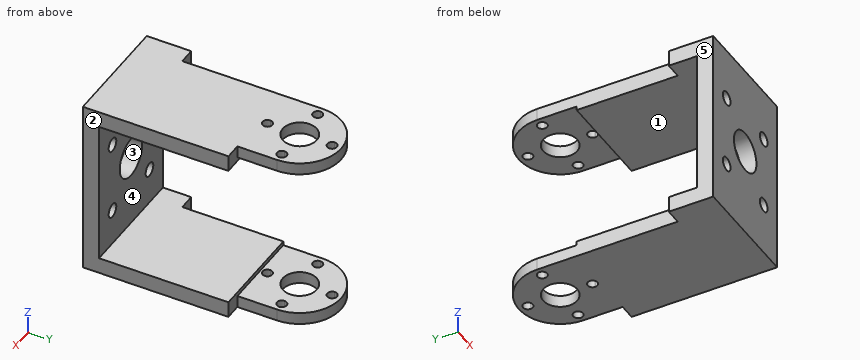
```python
from build123d import *

# Parameters (mm, degrees)
BOSS_EXTRUDE1_DEPTH      = 22
BOSS_EXTRUDE1_DEPTH_BACK = 22
SKETCH2_W                = 38
SKETCH2_H                = 20
CUT_EXTRUDE1_DEPTH       = 105.423416914
SKETCH3_W                = 7
SKETCH3_H                = 44
BOSS_EXTRUDE2_DEPTH      = 36
SKETCH5_W                = 34
SKETCH5_H                = 50
CUT_EXTRUDE3_DEPTH       = 109.047443283
SKETCH6_W                = 20.5
SKETCH6_H                = 54.25
CUT_EXTRUDE4_DEPTH       = 111.605436123
SKETCH20_W               = 28.5
SKETCH20_H               = 34
SKETCH20_R               = 1.7
SKETCH20_R_2             = 5
BOSS_EXTRUDE5_DEPTH      = 4
SKETCH21_W               = 3
SKETCH21_H               = 36
CUT_EXTRUDE12_DEPTH      = 66.777085676
SKETCH22_W               = 4
SKETCH22_H               = 25
CUT_EXTRUDE14_DEPTH      = 66.054784605
CUT_EXTRUDE15_DEPTH      = 57.367654732
CUT_EXTRUDE15_DEPTH_BACK = 57.367654732
SKETCH23_W               = 36
SKETCH23_H               = 32


with BuildPart() as part:
    # Sketch1 → Boss-Extrude1 (new, two sides: drawn at the far end of the back side and taken through both)
    with BuildSketch(Plane.XY.offset(-BOSS_EXTRUDE1_DEPTH_BACK)):
        with BuildLine():
            Line((10.25, -60), (10.25, 0))
            ThreePointArc((10.25, 0), (0, -10.25), (-10.25, 0))
            Line((-10.25, 0), (-10.25, -60))
            Line((-10.25, -60), (-10.25, -100))
            Line((-10.25, -100), (10.25, -100))
            Line((10.25, -100), (10.25, -60))
        make_face()
        with BuildLine():
            Line((10.25, 0), (9.2, 0))
            ThreePointArc((9.2, 0), (8.816088231, -0.879772698), (7.91, -1.196620241))
            ThreePointArc((7.91, -1.196620241), (5.656854249, -5.656854249), (1.196620241, -7.91))
            ThreePointArc((1.196620241, -7.91), (1.199154762, -7.954968281), (1.2, -8))
            ThreePointArc((1.2, -8), (-0.045031719, -9.199154762), (-1.196620241, -7.91))
            ThreePointArc((-1.196620241, -7.91), (-5.656854249, -5.656854249), (-7.91, -1.196620241))
            ThreePointArc((-7.91, -1.196620241), (-8.816088231, -0.879772698), (-9.2, 0))
            Line((-9.2, 0), (-10.25, 0))
            ThreePointArc((-10.25, 0), (0, -10.25), (10.25, 0))
        make_face()
        with BuildLine():
            ThreePointArc((7.91, -1.196620241), (7.120227302, -0.816088231), (6.8, 0))
            Line((6.8, 0), (4.2, 0))
            ThreePointArc((4.2, 0), (0, -4.2), (-4.2, 0))
            Line((-4.2, 0), (-6.8, 0))
            ThreePointArc((-6.8, 0), (-7.120227302, -0.816088231), (-7.91, -1.196620241))
            ThreePointArc((-7.91, -1.196620241), (-5.656854249, -5.656854249), (-1.196620241, -7.91))
            ThreePointArc((-1.196620241, -7.91), (0, -6.8), (1.196620241, -7.91))
            ThreePointArc((1.196620241, -7.91), (5.656854249, -5.656854249), (7.91, -1.196620241))
        make_face()
        with BuildLine():
            Line((4.2, 0), (6.8, 0))
            ThreePointArc((6.8, 0), (7.120227302, 0.816088231), (7.91, 1.196620241))
            ThreePointArc((7.91, 1.196620241), (5.656854249, 5.656854249), (1.196620241, 7.91))
            ThreePointArc((1.196620241, 7.91), (0, 6.8), (-1.196620241, 7.91))
            ThreePointArc((-1.196620241, 7.91), (-5.656854249, 5.656854249), (-7.91, 1.196620241))
            ThreePointArc((-7.91, 1.196620241), (-7.120227302, 0.816088231), (-6.8, 0))
            Line((-6.8, 0), (-4.2, 0))
            ThreePointArc((-4.2, 0), (0, 4.2), (4.2, 0))
        make_face()
        with BuildLine():
            ThreePointArc((7.91, 1.196620241), (8.816088231, 0.879772698), (9.2, 0))
            Line((9.2, 0), (10.25, 0))
            ThreePointArc((10.25, 0), (0, 10.25), (-10.25, 0))
            Line((-10.25, 0), (-9.2, 0))
            ThreePointArc((-9.2, 0), (-8.816088231, 0.879772698), (-7.91, 1.196620241))
            ThreePointArc((-7.91, 1.196620241), (-5.656854249, 5.656854249), (-1.196620241, 7.91))
            ThreePointArc((-1.196620241, 7.91), (-0.045031719, 9.199154762), (1.2, 8))
            ThreePointArc((1.2, 8), (1.199154762, 7.954968281), (1.196620241, 7.91))
            ThreePointArc((1.196620241, 7.91), (5.656854249, 5.656854249), (7.91, 1.196620241))
        make_face()
    extrude(amount=BOSS_EXTRUDE1_DEPTH + BOSS_EXTRUDE1_DEPTH_BACK)

    # Sketch2 → Cut-Extrude1 (cut, through all)
    with BuildSketch(Plane.ZY.offset(10.25)):
        with Locations((0, 0.25)):
            Rectangle(SKETCH2_W, SKETCH2_H)
    extrude(amount=-CUT_EXTRUDE1_DEPTH, mode=Mode.SUBTRACT)

    # Sketch3 → Boss-Extrude2 (add)
    with BuildSketch(Plane(origin=(0, -9.75, 0), x_dir=(1, 0, 0), z_dir=(0, 1, 0))):
        with Locations((-13.75, 0)):
            Rectangle(SKETCH3_W, SKETCH3_H)
        with Locations((13.75, 0)):
            Rectangle(SKETCH3_W, SKETCH3_H)
    extrude(amount=-BOSS_EXTRUDE2_DEPTH)

    # Sketch5 → Cut-Extrude3 (cut, through all)
    with BuildSketch(Plane.ZY.offset(17.25)):
        with Locations((0, -34.75)):
            Rectangle(SKETCH5_W, SKETCH5_H)
    extrude(amount=-CUT_EXTRUDE3_DEPTH, mode=Mode.SUBTRACT)

    # Sketch6 → Cut-Extrude4 (cut, through all)
    with BuildSketch(Plane.XY.offset(22)):
        with Locations((0, -72.875)):
            Rectangle(SKETCH6_W, SKETCH6_H)
    extrude(amount=-CUT_EXTRUDE4_DEPTH, mode=Mode.SUBTRACT)


with BuildPart() as cut_extrude4_piece_1:
    # of the separate pieces the step leaves, piece 1, a body of its own (cut_extrude4_pieces)
    add(part.part.solids().sort_by_distance((10.25, 0, -22))[0])



with BuildPart() as cut_extrude4_piece_2:
    # of the separate pieces the step leaves, piece 2, a body of its own (cut_extrude4_pieces)
    add(part.part.solids().sort_by_distance((17.25, -45.75, 22))[0])


with BuildPart() as cut_extrude4_piece_1_1:
    add(cut_extrude4_piece_1.part)

    add(cut_extrude4_piece_2.part)  # Boss-Extrude5 merges Cut-Extrude4 piece 2
    # Sketch20 → Boss-Extrude5 (add)
    with BuildSketch(Plane.XZ.offset(45.75)):
        Rectangle(SKETCH20_W, SKETCH20_H)
        with Locations(Location((-8.25, -9, 0), (0, 0, 270))):
            Circle(SKETCH20_R, mode=Mode.SUBTRACT)
        with Locations(Location((8.25, -9, 0), (0, 0, 270))):
            Circle(SKETCH20_R, mode=Mode.SUBTRACT)
        with Locations(Location((-8.25, 9, 0), (0, 0, 270))):
            Circle(SKETCH20_R, mode=Mode.SUBTRACT)
        with Locations(Location((0, 0, 0), (0, 0, 270))):
            Circle(SKETCH20_R_2, mode=Mode.SUBTRACT)
        with Locations(Location((8.25, 9, 0), (0, 0, 270))):
            Circle(SKETCH20_R, mode=Mode.SUBTRACT)
    extrude(amount=-BOSS_EXTRUDE5_DEPTH)

    # Sketch21 → Cut-Extrude12 (cut, through all)
    with BuildSketch(Plane(origin=(0, 0, -22), x_dir=(-1, 0, 0), z_dir=(0, 0, -1))):
        with Locations((-15.75, -27.75)):
            Rectangle(SKETCH21_W, SKETCH21_H)
        with Locations((15.75, -27.75)):
            Rectangle(SKETCH21_W, SKETCH21_H)
    extrude(amount=-CUT_EXTRUDE12_DEPTH, mode=Mode.SUBTRACT)

    # Sketch22 → Cut-Extrude14 (cut, through all)
    with BuildSketch(Plane(origin=(0, 0, -22), x_dir=(-1, 0, 0), z_dir=(0, 0, -1))):
        with Locations((12.25, -22.25)):
            Rectangle(SKETCH22_W, SKETCH22_H)
    extrude(amount=-CUT_EXTRUDE14_DEPTH, mode=Mode.SUBTRACT)

    # Sketch23 → Cut-Extrude15 (cut, two sides: drawn at the far end of the back side and taken through both)
    with BuildSketch(Plane.ZY.offset(10.25).offset(-CUT_EXTRUDE15_DEPTH_BACK)):
        with Locations((0, -25.75)):
            Rectangle(SKETCH23_W, SKETCH23_H)
    extrude(amount=CUT_EXTRUDE15_DEPTH + CUT_EXTRUDE15_DEPTH_BACK, mode=Mode.SUBTRACT)


solid = cut_extrude4_piece_1_1.part
```
Read the model definition and answer for the solid it produces. Units are mm, in the model's axes. Face numbers are marked on the shaded views. A direction names the side the tool comes from. Give positions to 0.01 mm unless a question says otherwise; leave off trailing zeros. Write each loop counter-clockwise with the first axis right and the second up, starting at its lowest first coordinate (ties: lowest second). Pieces come first, ordered by that corner, then holes. Notation, with made-up numbers: M -14.75,71.5 L -9.75,71.5 A36 cw -9.75,108.5 Z; hole C -39.5,-13 d5. An arc over 180 degrees is marked long. Put each result on its own line as item: value. Start each with the question number.
1. Consider line 1 along X through (y, z) = (-42.65, 9); line 2 along Z through (x, y) = (-4, -7); line 3 along Z through (x, y) = (-4.25, -37). Determine where each line is inside the solid, lowest interval first.
2. The part is cut by section D-D, the plane z = -9. Give the vertices of the cut face in (x, y), and give its area (3 significant figures).
3. For a pull along X with two mould halves and no side action, classify the marked faces 1, 2 and 3 as released by +X, released by -X, zero draft, split by the parting line, or undercut.
4. The part is cut by section B-B, the plane z = 0. Give the vertices of the cut face in (x, y), and give its area (3 significant figures).
5. The part is cut by section C-C, the plane x = 3.25. Give the vertices of the cut face in (y, z).
6. Which of the six approach directions +Z, -Z, +X, -X, +Y, -Y give full straight-line access (tool end or side, diameter ignored) to the marked faces 4 and 5?
7. Each of these flat-tipped pins is pushed along its axis until it touches: pin 1 Ø4 at (x, z) = (8.25, 9) entering from +Y; pin 2 Ø1.5 at (y, z) = (-3, 21) entering from +X; pin 3 Ø2 at (y, z) = (-10.5, 20.5) entering from -X. Where does it stop, or does it pass through?
8. The part is cut by section A-A, the plane y = -15.5. Give the vertices of the cut face in (x, z).
Final values:
1. line 1: x = -14.25 to -9.95, -6.55 to 6.55, 9.95 to 14.25
1. line 2: z = -22 to -19, 19 to 22
1. line 3: z = -22 to -18, 18 to 22
2. outline: M -14.25,-45.75 L -9.95,-45.75 L -9.95,-41.75 L -14.25,-41.75 Z; M -6.55,-45.75 L 6.55,-45.75 L 6.55,-41.75 L -6.55,-41.75 Z; M 9.95,-45.75 L 14.25,-45.75 L 14.25,-41.75 L 9.95,-41.75 Z
2. area: 86.8 mm²
3. face 1: zero draft
3. face 2: released by +X
3. face 3: undercut
4. outline: M -14.25,-45.75 L -5,-45.75 L -5,-41.75 L -14.25,-41.75 Z; M 5,-45.75 L 14.25,-45.75 L 14.25,-41.75 L 5,-41.75 Z
4. area: 74.0 mm²
5. outline: M -45.75,-22 L -2.66,-22 L -2.66,-19 L -9.75,-19 L -9.75,-18 L -41.75,-18 L -41.75,-3.8 L -45.75,-3.8 Z; M -45.75,3.8 L -41.75,3.8 L -41.75,18 L -9.75,18 L -9.75,19 L -2.66,19 L -2.66,22 L -45.75,22 Z; M 2.66,-22 L 9.72,-22 L 9.72,-19 L 2.66,-19 Z; M 2.66,19 L 9.72,19 L 9.72,22 L 2.66,22 Z
6. face 4: +X, -X, +Y
6. face 5: +Z, -Z, -X, +Y, -Y
7. pin 1: stops at y = -41.75
7. pin 2: stops at x = 10.25
7. pin 3: stops at x = -10.25
8. outline: M -10.25,-22 L 14.25,-22 L 14.25,-18 L -10.25,-18 Z; M -10.25,18 L 14.25,18 L 14.25,22 L -10.25,22 Z
